For this review, take the finished solid that the model builds, in its own axes (mm). Face numbers are marked on the shaded views. A direction names the side the tool comes from. Coordinates: 2 decimals unless noted, no trailing zeros. Loops run counter-clockwise (first coordinate to the right, second up) from the corner with the lowest first, then second, coordinate; pieces in that order, holes last.
1. Take a section at D-D, the plane x = 213.5. State the section outline as (y, z) points.
2. Mouldability with a two-part tool opening along X and no side actions: class the marked faces 1, 2 and 3 as pulls with the +X half, pulls with the -X half, needs draft (parallel to the pull), parting line crosses it, or undercut.
3. Clearance check with flat-ended pins moving along their axes: P1, Ø9.5, axis at x = 306.02, y = -10.34, coming from the -Z side; P2, Ø3, axis at x = 247.5, y = 147, coming from the +Z side; P3, Ø2, axis at y = 162.5, z = 145.5, coming from the +X side. State where each tip first meets the part, or that it passes through.
4. Take a section at C-C, the plane x = -136. State the section outline as (y, z) points, then the cut area to 3 significant figures.
5. Take a section at B-B, the plane z = 83. State the section outline as (x, y) points.
6. To check wall thickness, follow probe 1 along X at (y, z) = (116, 76.5); probe 2 along Y at (x, z) = (-223, 53); probe 3 along Z at (x, y) = (334.5, 163.5). State the ranges of each line that lie inside material, in increasing order.
7. Take a section at A-A, the plane x = 67. State the section outline as (y, z) points, then the cut area to 3 significant figures.
8. Machinability: for the marked faces 4 and 5, which of the approach directions +Z, -Z, +X, -X, +Y, -Y give a long, thin tool a straight path to every point of the face, cutting with its end or side? Answer none if there is none.
```python
from build123d import *

# Parameters (mm, degrees)
SKETCH1_W                = 760
SKETCH1_H                = 350
BOSS_EXTRUDE1_DEPTH      = 38
SKETCH2_R                = 65
SKETCH2_R_2              = 55
SKETCH2_R_3              = 45
CUT_EXTRUDE1_DEPTH       = 473.628796964
CUT_EXTRUDE3_DEPTH       = 473.628796964
SKETCH5_R                = 75
SKETCH5_R_2              = 3
SKETCH5_R_3              = 70
SKETCH5_R_4              = 40
CUT_EXTRUDE7_DEPTH       = 7
SKETCH7_R                = 3
CUT_EXTRUDE8_DEPTH       = 473.628796964
SKETCH8_W                = 760
SKETCH8_H                = 350
CUT_EXTRUDE9_DEPTH       = 18
SKETCH9_OUTSIDE_W        = 929.392
SKETCH9_OUTSIDE_H        = 519.392
CUT_EXTRUDE10_DEPTH      = 472.523042618
BOSS_EXTRUDE2_DEPTH      = 194
FILLET1_R                = 10
SKETCH12_R               = 40
SKETCH12_R_2             = 20
SKETCH12_R_3             = 3
BOSS_EXTRUDE4_DEPTH      = 7
BOSS_EXTRUDE4_DEPTH_BACK = 2
SKETCH13_R               = 3
BOSS_EXTRUDE8_DEPTH      = 20
SKETCH11_R               = 80
SKETCH11_R_2             = 3
CUT_EXTRUDE11_DEPTH      = 7
SKETCH15_R               = 3
CUT_EXTRUDE12_DEPTH      = 518.42630366
FILLET2_R                = 30


with BuildPart() as part:
    # Sketch1 → Boss-Extrude1 (new body)
    with BuildSketch(Plane.XY):
        with Locations((42.843137255, 32.696078431)):
            Rectangle(SKETCH1_W, SKETCH1_H)
    extrude(amount=BOSS_EXTRUDE1_DEPTH)

    # Sketch2 → Cut-Extrude1 (cut, through all)
    with BuildSketch(Plane.XY.offset(38)):
        with Locations((245.403137255, 24.656078431)):
            Circle(SKETCH2_R)
        with Locations((91.403137255, 24.656078431)):
            Circle(SKETCH2_R_2)
        with Locations((-54.006862745, 24.656078431)):
            Circle(SKETCH2_R_3)
    extrude(amount=-CUT_EXTRUDE1_DEPTH, mode=Mode.SUBTRACT)

    # Sketch3 → Cut-Extrude3 (cut, through all)
    with BuildSketch(Plane.XY.offset(38)):
        with BuildLine():
            ThreePointArc((-211.086862745, 24.656078431), (-191.086862745, 4.656078431), (-171.086862745, 24.656078431))
            Line((-171.086862745, 24.656078431), (-191.086862745, 24.656078431))
            Line((-191.086862745, 24.656078431), (-211.086862745, 24.656078431))
        make_face()
        with BuildLine():
            Line((-191.086862745, 24.656078431), (-171.086862745, 24.656078431))
            ThreePointArc((-171.086862745, 24.656078431), (-191.086862745, 44.656078431), (-211.086862745, 24.656078431))
            Line((-211.086862745, 24.656078431), (-191.086862745, 24.656078431))
        make_face()
    extrude(amount=-CUT_EXTRUDE3_DEPTH, mode=Mode.SUBTRACT)

    # Sketch5 → Cut-Extrude7 (cut)
    with BuildSketch(Plane(origin=(0, 0, 0), x_dir=(-1, 0, 0), z_dir=(0, 0, -1))):
        with Locations((54.006862745, 24.656078431)):
            Circle(SKETCH5_R)
        with Locations((54.006862745, 84.656078431)):
            Circle(SKETCH5_R_2, mode=Mode.SUBTRACT)
        with Locations((105.968386972, -5.343921569)):
            Circle(SKETCH5_R_2, mode=Mode.SUBTRACT)
        with Locations((2.045338518, -5.343921569)):
            Circle(SKETCH5_R_2, mode=Mode.SUBTRACT)
        with Locations((-91.403137255, 24.656078431)):
            Circle(SKETCH5_R_3)
        with Locations((-91.403137255, 84.656078431)):
            Circle(SKETCH5_R_2, mode=Mode.SUBTRACT)
        with Locations((-39.441613028, -5.343921569)):
            Circle(SKETCH5_R_2, mode=Mode.SUBTRACT)
        with Locations((-143.364661482, -5.343921569)):
            Circle(SKETCH5_R_2, mode=Mode.SUBTRACT)
        with Locations((191.086862745, 24.656078431)):
            Circle(SKETCH5_R_4)
        with Locations((191.086862745, 54.656078431)):
            Circle(SKETCH5_R_2, mode=Mode.SUBTRACT)
        with Locations((217.067624859, 9.656078431)):
            Circle(SKETCH5_R_2, mode=Mode.SUBTRACT)
        with Locations((165.106100632, 9.656078431)):
            Circle(SKETCH5_R_2, mode=Mode.SUBTRACT)
    extrude(amount=-CUT_EXTRUDE7_DEPTH, mode=Mode.SUBTRACT)

    # Sketch7 → Cut-Extrude8 (cut, through all)
    with BuildSketch(Plane(origin=(0, 0, 0), x_dir=(-1, 0, 0), z_dir=(0, 0, -1))):
        with Locations((-91.403137255, 84.656078431)):
            Circle(SKETCH7_R)
        with Locations((-143.364661482, -5.343921569)):
            Circle(SKETCH7_R)
        with Locations((-39.441613028, -5.343921569)):
            Circle(SKETCH7_R)
        with Locations((2.045338518, -5.343921569)):
            Circle(SKETCH7_R)
        with Locations((54.006862745, 84.656078431)):
            Circle(SKETCH7_R)
        with Locations((105.968386972, -5.343921569)):
            Circle(SKETCH7_R)
        with Locations((191.086862745, 54.656078431)):
            Circle(SKETCH7_R)
        with Locations((165.106100632, 9.656078431)):
            Circle(SKETCH7_R)
        with Locations((217.067624859, 9.656078431)):
            Circle(SKETCH7_R)
    extrude(amount=-CUT_EXTRUDE8_DEPTH, mode=Mode.SUBTRACT)

    # Sketch8 → Cut-Extrude9 (cut)
    with BuildSketch(Plane.XY.offset(38)):
        with Locations((42.843137255, 32.696078431)):
            Rectangle(SKETCH8_W, SKETCH8_H)
    extrude(amount=-CUT_EXTRUDE9_DEPTH, mode=Mode.SUBTRACT)

    # Sketch9 outside → Cut-Extrude10 (cut, through all)
    with BuildSketch(Plane.XY.offset(20)):
        with Locations((42.843, 32.696)):
            Rectangle(SKETCH9_OUTSIDE_W, SKETCH9_OUTSIDE_H)
        with BuildLine():
            Line((-277.156862745, 207.696078431), (362.843137255, 207.696078431))
            ThreePointArc((362.843137255, 207.696078431), (405.269544126, 190.122485303), (422.843137255, 147.696078431))
            Line((422.843137255, 147.696078431), (422.843137255, -82.303921569))
            ThreePointArc((422.843137255, -82.303921569), (405.269544126, -124.73032844), (362.843137255, -142.303921569))
            Line((362.843137255, -142.303921569), (-277.156862745, -142.303921569))
            ThreePointArc((-277.156862745, -142.303921569), (-319.583269616, -124.73032844), (-337.156862745, -82.303921569))
            Line((-337.156862745, -82.303921569), (-337.156862745, 147.696078431))
            ThreePointArc((-337.156862745, 147.696078431), (-319.583269616, 190.122485303), (-277.156862745, 207.696078431))
        make_face(mode=Mode.SUBTRACT)
    extrude(amount=-CUT_EXTRUDE10_DEPTH, mode=Mode.SUBTRACT)

    # Sketch10 → Boss-Extrude2 (add)
    with BuildSketch(Plane.XY.offset(20)):
        with BuildLine():
            Line((-277.156862745, 207.696078431), (362.843137255, 207.696078431))
            ThreePointArc((362.843137255, 207.696078431), (405.269544126, 190.122485303), (422.843137255, 147.696078431))
            Line((422.843137255, 147.696078431), (422.843137255, -82.303921569))
            ThreePointArc((422.843137255, -82.303921569), (405.269544126, -124.73032844), (362.843137255, -142.303921569))
            Line((362.843137255, -142.303921569), (-277.156862745, -142.303921569))
            ThreePointArc((-277.156862745, -142.303921569), (-319.583269616, -124.73032844), (-337.156862745, -82.303921569))
            Line((-337.156862745, -82.303921569), (-337.156862745, 147.696078431))
            ThreePointArc((-337.156862745, 147.696078431), (-319.583269616, 190.122485303), (-277.156862745, 207.696078431))
        make_face()
        with BuildLine():
            Line((-245.441133993, 175.980349679), (331.127408502, 175.980349679))
            ThreePointArc((331.127408502, 175.980349679), (373.553815374, 158.40675655), (391.127408502, 115.980349679))
            Line((391.127408502, 115.980349679), (391.127408502, -50.588192816))
            ThreePointArc((391.127408502, -50.588192816), (373.553815374, -93.014599687), (331.127408502, -110.588192816))
            Line((331.127408502, -110.588192816), (-245.441133993, -110.588192816))
            ThreePointArc((-245.441133993, -110.588192816), (-287.867540864, -93.014599687), (-305.441133993, -50.588192816))
            Line((-305.441133993, -50.588192816), (-305.441133993, 115.980349679))
            ThreePointArc((-305.441133993, 115.980349679), (-287.867540864, 158.40675655), (-245.441133993, 175.980349679))
        make_face(mode=Mode.SUBTRACT)
    extrude(amount=BOSS_EXTRUDE2_DEPTH)

    # Fillet1
    fillet1_edges = [part.edges().sort_by_distance(p)[0] for p in [
        (-287.867540864, -93.014599687, 20),
        (42.843137255, -110.588192816, 20),
        (373.553815374, -93.014599687, 20),
        (391.127408502, 32.696078431, 20),
        (373.553815374, 158.40675655, 20),
        (42.843137255, 175.980349679, 20),
        (-287.867540864, 158.40675655, 20),
        (-305.441133993, 32.696078431, 20),
    ]]
    fillet(fillet1_edges, radius=FILLET1_R)

    # Sketch12 → Boss-Extrude4 (add, two sides)
    with BuildSketch(Plane(origin=(0, 0, 7), x_dir=(-1, 0, 0), z_dir=(0, 0, -1))) as boss_extrude4_sk:
        with Locations((191.086862745, 24.656078431)):
            Circle(SKETCH12_R)
        with Locations(Location((191.086862745, 24.656078431, 0), (0, 0, 180))):
            Circle(SKETCH12_R_2, mode=Mode.SUBTRACT)
        with Locations((191.086862745, 54.656078431)):
            Circle(SKETCH12_R_3, mode=Mode.SUBTRACT)
        with Locations((165.106100632, 9.656078431)):
            Circle(SKETCH12_R_3, mode=Mode.SUBTRACT)
        with Locations((217.067624859, 9.656078431)):
            Circle(SKETCH12_R_3, mode=Mode.SUBTRACT)
    extrude(amount=BOSS_EXTRUDE4_DEPTH)
    extrude(boss_extrude4_sk.sketch, amount=-BOSS_EXTRUDE4_DEPTH_BACK)

    # Sketch13 → Boss-Extrude8 (add)
    with BuildSketch(Plane(origin=(0, 0, 0), x_dir=(-1, 0, 0), z_dir=(0, 0, -1))):
        with Locations((191.086862745, 54.656078431)):
            Circle(SKETCH13_R)
        with Locations((217.067624859, 9.656078431)):
            Circle(SKETCH13_R)
        with Locations((165.106100632, 9.656078431)):
            Circle(SKETCH13_R)
    extrude(amount=-BOSS_EXTRUDE8_DEPTH)

    # Sketch11 → Cut-Extrude11 (cut)
    with BuildSketch(Plane(origin=(0, 0, 0), x_dir=(-1, 0, 0), z_dir=(0, 0, -1))):
        with Locations((-245.403137255, 24.656078431)):
            Circle(SKETCH11_R)
        with Locations((-245.403137255, 94.656078431)):
            Circle(SKETCH11_R_2, mode=Mode.SUBTRACT)
        with Locations((-184.78135899, -10.343921569)):
            Circle(SKETCH11_R_2, mode=Mode.SUBTRACT)
        with Locations((-306.02491552, -10.343921569)):
            Circle(SKETCH11_R_2, mode=Mode.SUBTRACT)
    extrude(amount=-CUT_EXTRUDE11_DEPTH, mode=Mode.SUBTRACT)

    # Sketch15 → Cut-Extrude12 (cut, through all)
    with BuildSketch(Plane(origin=(0, 0, 0), x_dir=(-1, 0, 0), z_dir=(0, 0, -1))):
        with Locations((-245.403137255, 94.656078431)):
            Circle(SKETCH15_R)
        with Locations((-306.02491552, -10.343921569)):
            Circle(SKETCH15_R)
        with Locations((-184.78135899, -10.343921569)):
            Circle(SKETCH15_R)
    extrude(amount=-CUT_EXTRUDE12_DEPTH, mode=Mode.SUBTRACT)

    # Fillet2
    fillet2_edges = [part.edges().sort_by_distance(p)[0] for p in [
        (-337.156862745, 32.696078431, 0),
        (42.843137255, 207.696078431, 0),
        (422.843137255, 32.696078431, 0),
        (42.843137255, -142.303921569, 0),
        (-319.583269616, -124.73032844, 0),
        (405.269544126, -124.73032844, 0),
        (405.269544126, 190.122485303, 0),
        (-319.583269616, 190.122485303, 0),
    ]]
    fillet(fillet2_edges, radius=FILLET2_R)


solid = part.part
```
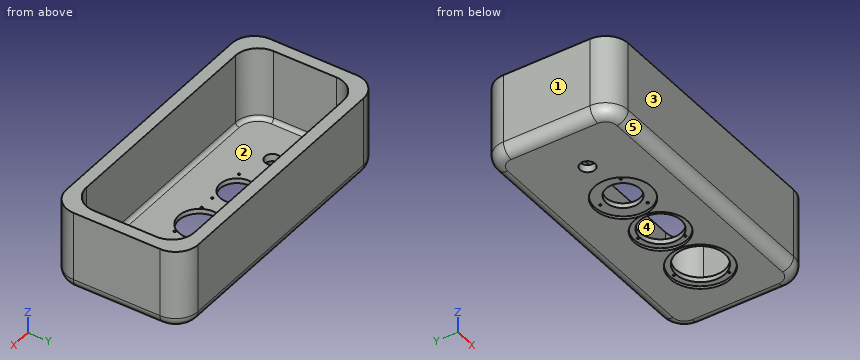
Results list:
1. outline: (-142.3, 30) arc R30 ccw to (-112.3, 0) - (-48.71, 0) - (-48.71, 7) - (-31.98, 7) - (-31.98, 20) - (-100.59, 20) arc R10 cw to (-110.59, 30) - (-110.59, 214) - (-142.3, 214) - close; (81.29, 7) - (98.02, 7) - (98.02, 0) - (177.7, 0) arc R30 ccw to (207.7, 30) - (207.7, 214) - (175.98, 214) - (175.98, 30) arc R10 cw to (165.98, 20) - (81.29, 20) - close
2. face 1: pulls with the -X half
2. face 2: undercut
2. face 3: needs draft
3. P1: stops at z = 7
3. P2: stops at z = 20
3. P3: stops at x = 421.23
4. outline: (-142.3, 30) arc R30 ccw to (-112.3, 0) - (177.7, 0) arc R30 ccw to (207.7, 30) - (207.7, 214) - (175.98, 214) - (175.98, 30) arc R10 cw to (165.98, 20) - (-100.59, 20) arc R10 cw to (-110.59, 30) - (-110.59, 214) - (-142.3, 214) - close
4. area: 19,000 mm2
5. outline: (-337.16, -82.3) arc R60 ccw to (-277.16, -142.3) - (362.84, -142.3) arc R60 ccw to (422.84, -82.3) - (422.84, 147.7) arc R60 ccw to (362.84, 207.7) - (-277.16, 207.7) arc R60 ccw to (-337.16, 147.7) - close; hole (-305.44, -50.59) arc R60 ccw to (-245.44, -110.59) - (331.13, -110.59) arc R60 ccw to (391.13, -50.59) - (391.13, 115.98) arc R60 ccw to (331.13, 175.98) - (-245.44, 175.98) arc R60 ccw to (-305.44, 115.98) - close
6. probe 1: x = -337.16 to -305.44, 391.13 to 422.84
6. probe 2: y = -142.3 to -110.59, 175.98 to 207.7
6. probe 3: z = 0 to 20
7. outline: (-142.3, 30) arc R30 ccw to (-112.3, 0) - (-40.95, 0) - (-40.95, 7) - (-24.63, 7) - (-24.63, 20) - (-100.59, 20) arc R10 cw to (-110.59, 30) - (-110.59, 214) - (-142.3, 214) - close; (73.95, 7) - (90.26, 7) - (90.26, 0) - (177.7, 0) arc R30 ccw to (207.7, 30) - (207.7, 214) - (175.98, 214) - (175.98, 30) arc R10 cw to (165.98, 20) - (73.95, 20) - close
7. area: 16,800 mm2
8. face 4: +Z
8. face 5: -Z, +X, -X, -Y
